Part model, mm, in its own coordinate system. A direction names the side the tool comes from. Give positions to 0.01 mm unless a question says otherwise; leave off trailing zeros. Write each loop counter-clockwise with the first axis right and the second up, starting at its lowest first coordinate (ties: lowest second). Pieces come first, ordered by that corner, then holes. Notation, with made-up numbers: M 50.25,9.5 L 56.25,9.5 A9 cw 56.25,17.5 Z; hole C -21.5,88 d7. An arc over 180 degrees is marked long. Use CSV: the item, a comma, the result in double quotes. Start each with the question number.
Item 1: Cut at C-C (x = 54.5). List the corners of the cut face in (y, z), then the cut area to 3 significant figures.
Item 2: Mould opens along X. For faces 6 (the cylindrical face through (102.9, -2.5, 0.1)), 7 (the cylindrical face through (106.5, 0, -1.5)), 8 (the flat face through (100, -1, 2)) say: released by +X, released by -X, zero draft, split by the parting line, or undercut.
Item 3: Which spindle directions (+Z, -Z, +X, -X, +Y, -Y) get a long thin tool onto all of the face, cutting with end or side? Do faces 1 (the cylindrical face through (49.3, -1.5, 0.07)), 2 (the flat face through (106, 0, 2)), 3 (the cylindrical face through (106.5, 0, 1.5)), 4 (the flat face through (106, 0, 1)), 5 (the flat face through (106, 0, -2)). Say none if no direction does.
Item 4: Drill centre lines: line 1 (Z direction, x = 69.5, y = 0); line 2 (Y direction, x = 51.5, z = -0.25); line 3 (X direction, y = 2.05, z = -0.5). Where is each one in solid material? Low to high. Write a range as [from, to].
Item 5: Pin check, flat tips, straight feed: pin 1 (2.5 mm diameter, centred on y = 0, z = 0, fed in from -X); pin 2 (1 mm diameter, centred on x = 28, y = 1.5, fed in from -Z); pin 3 (1 mm diameter, centred on y = -1.5, z = -1.5, fed in from +X). Stop position of each tip, or through.
Item 6: Cut at A-A (y = 0). List the corners of the cut face in (x, z).
Item 7: Cut at B-B (z = 0). List the corners of the cut face in (x, y), then the cut area to 4 significant figures.
from build123d import *

# Parameters (mm, degrees)
F0_R     = 2
F0_R_2   = 1.5
F1_DEPTH = 100
F2_R     = 2.5
F2_R_2   = 2
F2_R_3   = 1.5
F3_DEPTH = 10
F4_R     = 2.5
F5_W     = 10
F5_H     = 2
F6_DEPTH = 5
F7_R     = 1
F8_DEPTH = 4.501


with BuildPart() as f1:
    # F0 (on Right) → F1 (new body)
    with BuildSketch(Plane.YZ):
        Circle(F0_R)
        Circle(F0_R_2, mode=Mode.SUBTRACT)
    extrude(amount=F1_DEPTH)

    # F2 (on face) → F3 (join)
    with BuildSketch(Plane.YZ.offset(100)):
        Circle(F2_R)
        Circle(F2_R_2, mode=Mode.SUBTRACT)
        Circle(F2_R_2)
        Circle(F2_R_3, mode=Mode.SUBTRACT)
        Circle(F2_R_3)
    extrude(amount=F3_DEPTH)

    # F4
    f4_edges = [f1.edges().sort_by_distance(p)[0] for p in [
        (110, -2.5, 0),
    ]]
    fillet(f4_edges, radius=F4_R)

    # F5 (on Front) → F6 (cut, symmetric)
    with BuildSketch(Plane.XZ):
        with Locations((109.5, 3)):
            Rectangle(F5_W, F5_H)
        with Locations((109.5, 0)):
            Rectangle(F5_W, F5_H)
        with Locations((109.5, -3)):
            Rectangle(F5_W, F5_H)
    extrude(amount=F6_DEPTH, both=True, mode=Mode.SUBTRACT)

    # F7 (on face) → F8 (cut, through all)
    with BuildSketch(Plane.XY.offset(2)):
        with Locations((107.5, 0)):
            Circle(F7_R)
    extrude(amount=-F8_DEPTH, mode=Mode.SUBTRACT)


solid = f1.part
Worked answers:
1,outline,"C 0,0 d4; hole C 0,0 d3"
1,area,"5.50 mm^2"
2,face 6,"zero draft"
2,face 7,"undercut"
2,face 8,"released by -X"
3,face 1,"-X"
3,face 2,"+Z, +X, +Y, -Y"
3,face 3,"+Z, -Z"
3,face 4,"+X, +Y, -Y"
3,face 5,"-Z, +X, +Y, -Y"
4,line 1,"z = [-2, -1.5], [1.5, 2]"
4,line 2,"y = [-1.98, -1.48], [1.48, 1.98]"
4,line 3,"x = [100, 104.5]"
5,pin 1,"stops at x = 100"
5,pin 2,"stops at z = -1.73"
5,pin 3,"stops at x = 109.4"
6,outline,"M 0,-2 L 100,-2 L 100,-2.5 L 104.5,-2.5 L 104.5,-2 L 106.5,-2 L 106.5,-1 L 104.5,-1 L 104.5,1 L 106.5,1 L 106.5,2 L 104.5,2 L 104.5,2.5 L 100,2.5 L 100,2 L 0,2 L 0,1.5 L 100,1.5 L 100,-1.5 L 0,-1.5 Z; M 108.5,-2 L 109,-2 A2.5 ccw 109.79,-1 L 108.5,-1 Z; M 108.5,1 L 109.79,1 A2.5 ccw 109,2 L 108.5,2 Z"
7,outline,"M 0,-2 L 100,-2 L 100,-2.5 L 104.5,-2.5 L 104.5,2.5 L 100,2.5 L 100,2 L 0,2 L 0,1.5 L 100,1.5 L 100,-1.5 L 0,-1.5 Z"
7,area,"122.5 mm^2"
